```python
from build123d import *

# Parameters (mm, degrees)
SKETCH_8_R          = 1
CUT_EXTRUDE_1_DEPTH = 31.8
SKETCH_9_W          = 0.43
SKETCH_9_H          = 0.4
HOLE_WIZARD_M3_2_D  = 2.5
SKETCH_13_R         = 11.79
CUT_EXTRUDE_2_DEPTH = 1.5
FILLET_1_R          = 1


with BuildPart() as part:
    # 草图3 → 旋转-薄壁1 (revolve)
    with BuildSketch(Plane.XY):
        Polygon((3.225, -1.7), (3.225, 0), (12.2, 0), (12.2, 30.8), (11.55, 30.8), (11.55, 0.65), (2.575, 0.65), (2.575, -1.7), align=None)
    revolve(axis=Axis((0, -2.280125191, 0), (0, 1, 0)))

    # 草图8 → 切除-拉伸1 (cut, through all)
    with BuildSketch(Plane.XZ):
        with Locations((-8.5, 0)):
            Circle(SKETCH_8_R)
        with Locations((8.5, 0)):
            Circle(SKETCH_8_R)
    extrude(amount=-CUT_EXTRUDE_1_DEPTH, mode=Mode.SUBTRACT)

    # 草图9 → 旋转-薄壁2 (revolve)
    with BuildSketch(Plane.XY):
        with Locations((-9.715, 0.85)):
            Rectangle(SKETCH_9_W, SKETCH_9_H)
    revolve(axis=Axis((-8.5, 2.007130547, 0), (0, -1, 0)))

    # M3 螺纹孔2 (through all)
    with Locations(Plane(origin=(0, 0, 0), x_dir=(-1, 0, 0), z_dir=(0, -1, 0))):
        with Locations((8.5, 0), (-8.5, 0)):
            Hole(HOLE_WIZARD_M3_2_D / 2)

    # 草图13 → 切除-拉伸2 (cut)
    with BuildSketch(Plane(origin=(0, 30.8, 0), x_dir=(1, 0, 0), z_dir=(0, 1, 0))):
        Circle(SKETCH_13_R)
    extrude(amount=-CUT_EXTRUDE_2_DEPTH, mode=Mode.SUBTRACT)

    # 圆角1
    fillet_1_edges = [part.edges().sort_by_distance(p)[0] for p in [
        (-12.2, 0, 0),
    ]]
    fillet(fillet_1_edges, radius=FILLET_1_R)


solid = part.part
```
For this review, take the finished solid that the model builds, in its own axes (mm). A direction names the side the tool comes from. Coordinates: 2 decimals unless noted, no trailing zeros. Loops run counter-clockwise (first coordinate to the right, second up) from the corner with the lowest first, then second, coordinate; pieces in that order, holes last. Notation, with made-up numbers: (12.25, 20.25) - (60.25, 20.25) arc R12 cw to (60.25, 40.25) - close; hole circle Ø9 at (-2.5, -26.75). An arc over 180 degrees is marked (long way). Use one line per item in the form item = value. Start each with the question number.
1) Draft analysis for pull direction Z (two halves, no side actions). For faces 1 (the face through (-0.7, -0.84, 3.15)), 2 (the face through (0, 0.65, -3)), 3 (the face through (0, -1.7, 3)), state which applies: released by +Z, released by -Z, zero draft, split by the parting line, or undercut.
2) Take a section at A-A (x = 0). State the section outline as (y, z) points (3 decimals), plus the area to 3 significant figures.
3) To check wall thickness, follow probe 1 along Z at (x, y) = (-8.5, 0.7); probe 2 along Z at (x, y) = (0, 10); probe 3 along Z at (x, y) = (0, 29.75). State the ranges of each line that lie inside material, in increasing order. Write a range as from..to.
4) Take a section at C-C (y = 20). State the section outline as (x, z) points.
5) For pin 1 (1 mm diameter, centred on x = -4, y = 17.5, fed in from -Z); pin 2 (4 mm diameter, centred on x = 7, z = -4.5, fed in from +Y); pin 3 (12 mm diameter, centred on x = -0.5, z = 0, fed in from +Y); pin 4 (14 mm diameter, centred on x = 0, z = 0, fed in from -Y), all flat-tipped, find the tip position at first contact; note any pin that passes through.
6) For faces 4 (the face through (-2, 0, -3)), 5 (the face through (7.25, 0.33, -0.05)), 6 (the face through (-2.6, 30.1, 11.5)), list the 3-axis set-ups (+Z, -Z, +X, -X, +Y, -Y) from which the entire face can be reached by the end or side of a thin tool; tool diameter is ignored.
7) Take a section at B-B (z = 0). State how many separate pieces and enclosed holes the cut face has, plus the area to 3 significant figures.
From the geometry:
q1.face_1 = split by the parting line
q1.face_2 = undercut
q1.face_3 = zero draft
q2.outline = (-1.7, -3.225) - (0, -3.225) - (0, -11.2) arc R1 ccw to (1, -12.2) - (30.8, -12.2) - (30.8, -11.79) - (29.3, -11.79) - (29.3, -11.55) - (0.65, -11.55) - (0.65, -2.575) - (-1.7, -2.575) - close; (-1.7, 2.575) - (0.65, 2.575) - (0.65, 11.55) - (29.3, 11.55) - (29.3, 11.79) - (30.8, 11.79) - (30.8, 12.2) - (1, 12.2) arc R1 ccw to (0, 11.2) - (0, 3.225) - (-1.7, 3.225) - close
q2.area = 52.8 mm2
q3.probe_1 = -8.69..-7.82, -1.43..-1.25, 1.25..1.43, 7.82..8.69
q3.probe_2 = -12.2..-11.55, 11.55..12.2
q3.probe_3 = -12.2..-11.79, 11.79..12.2
q4.outline = circle Ø24.4 at (0, 0); hole circle Ø23.1 at (0, 0)
q5.pin_1 = -11.69
q5.pin_2 = 0.65
q5.pin_3 = 0.65
q5.pin_4 = -1.7
q6.face_4 = -Y
q6.face_5 = +Y, -Y
q6.face_6 = +Y
q7.separate_pieces = 4
q7.enclosed_holes = 0
q7.area = 49.7 mm2
